```python
from build123d import *

# Parameters (mm, degrees)
SKETCH1_W                          = 101.6
SKETCH1_H                          = 31.75
BOSS_EXTRUDE1_DEPTH                = 3.175
CUT_EXTRUDE1_REACH                 = 55.6
SKETCH2_R                          = 1.63195
SKETCH2_R_2                        = 6.35
TAP_DRILL_FOR_6_32_TAP1_AT_2_COUNT = 2
TAP_DRILL_FOR_6_32_TAP1_AT_2_PITCH = 79.375
TAP_DRILL_FOR_6_32_TAP1_AT_3_COUNT = 2
TAP_DRILL_FOR_6_32_TAP1_AT_3_PITCH = 47.625


with BuildPart() as part:
    # Sketch1 → Boss-Extrude1 (new, symmetric)
    with BuildSketch(Plane(origin=(0, 0, 0), x_dir=(0, 0, -1), z_dir=(1, 0, 0))):
        Rectangle(SKETCH1_W, SKETCH1_H)
    extrude(amount=BOSS_EXTRUDE1_DEPTH, both=True)

    # Sketch2 → Cut-Extrude1 (cut, up to next)
    with BuildSketch(Plane(origin=(3.175, 0, 0), x_dir=(0, 0, -1), z_dir=(1, 0, 0)), mode=Mode.PRIVATE) as cut_extrude1_sk1:
        with Locations((-16.764, 8.255)):
            Circle(SKETCH2_R)
    cut_extrude1_tool1 = extrude(cut_extrude1_sk1.sketch, amount=-CUT_EXTRUDE1_REACH, mode=Mode.PRIVATE) & part.part
    # Sketch2 → Cut-Extrude1 (cut, up to next)
    with BuildSketch(Plane(origin=(3.175, 0, 0), x_dir=(0, 0, -1), z_dir=(1, 0, 0)), mode=Mode.PRIVATE) as cut_extrude1_sk2:
        with Locations((-16.764, -12.7)):
            Circle(SKETCH2_R)
    cut_extrude1_tool2 = extrude(cut_extrude1_sk2.sketch, amount=-CUT_EXTRUDE1_REACH, mode=Mode.PRIVATE) & part.part
    # Sketch2 → Cut-Extrude1 (cut, up to next)
    with BuildSketch(Plane(origin=(3.175, 0, 0), x_dir=(0, 0, -1), z_dir=(1, 0, 0)), mode=Mode.PRIVATE) as cut_extrude1_sk3:
        with Locations((40.005, -12.7)):
            Circle(SKETCH2_R)
    cut_extrude1_tool3 = extrude(cut_extrude1_sk3.sketch, amount=-CUT_EXTRUDE1_REACH, mode=Mode.PRIVATE) & part.part
    # Sketch2 → Cut-Extrude1 (cut, up to next)
    with BuildSketch(Plane(origin=(3.175, 0, 0), x_dir=(0, 0, -1), z_dir=(1, 0, 0)), mode=Mode.PRIVATE) as cut_extrude1_sk4:
        with Locations((40.005, 8.255)):
            Circle(SKETCH2_R)
    cut_extrude1_tool4 = extrude(cut_extrude1_sk4.sketch, amount=-CUT_EXTRUDE1_REACH, mode=Mode.PRIVATE) & part.part
    # Sketch2 → Cut-Extrude1 (cut, up to next)
    with BuildSketch(Plane(origin=(3.175, 0, 0), x_dir=(0, 0, -1), z_dir=(1, 0, 0)), mode=Mode.PRIVATE) as cut_extrude1_sk5:
        with Locations((-4.064, -2.2225)):
            Circle(SKETCH2_R_2)
    cut_extrude1_tool5 = extrude(cut_extrude1_sk5.sketch, amount=-CUT_EXTRUDE1_REACH, mode=Mode.PRIVATE) & part.part
    add(cut_extrude1_tool1.solids().sort_by_distance((3.175, 8.255, 16.764))[0], mode=Mode.SUBTRACT)
    add(cut_extrude1_tool2.solids().sort_by_distance((3.175, -12.7, 16.764))[0], mode=Mode.SUBTRACT)
    add(cut_extrude1_tool3.solids().sort_by_distance((3.175, -12.7, -40.005))[0], mode=Mode.SUBTRACT)
    add(cut_extrude1_tool4.solids().sort_by_distance((3.175, 8.255, -40.005))[0], mode=Mode.SUBTRACT)
    add(cut_extrude1_tool5.solids().sort_by_distance((3.175, -2.2225, 4.064))[0], mode=Mode.SUBTRACT)

    # Sketch5 → Tap Drill for #6-32 Tap1 (revolve, cut)
    with BuildSketch(Plane(origin=(0, 15.875, 44.45), x_dir=(0, 0, 1), z_dir=(1, 0, 0))):
        Polygon((0, 0), (0, 13.51269403), (1.35255, 12.7), (1.35255, 0), align=None)
    tap_drill_for_6_32_tap1 = revolve(axis=Axis((0, 22.225, 44.45), (0, -1, 0)), mode=Mode.SUBTRACT)

    # Tap Drill for #6-32 Tap1 at 2: Tap Drill for #6-32 Tap1 ×2
    with Locations(*[(0, 0, -i * TAP_DRILL_FOR_6_32_TAP1_AT_2_PITCH) for i in range(1, TAP_DRILL_FOR_6_32_TAP1_AT_2_COUNT)]):
        add(tap_drill_for_6_32_tap1, mode=Mode.SUBTRACT)

    # Tap Drill for #6-32 Tap1 at 3: Tap Drill for #6-32 Tap1 ×2
    with Locations(*[(0, 0, -i * TAP_DRILL_FOR_6_32_TAP1_AT_3_PITCH) for i in range(1, TAP_DRILL_FOR_6_32_TAP1_AT_3_COUNT)]):
        add(tap_drill_for_6_32_tap1, mode=Mode.SUBTRACT)

    # Mirror1: Tap Drill for #6-32 Tap1 across plane
    add(tap_drill_for_6_32_tap1.mirror(Plane.ZX), mode=Mode.SUBTRACT)

    # Mirror1 copy 1 sketch → Mirror1 copy 1 (revolve, cut)
    with BuildSketch(Plane(origin=(0, -15.875, -34.925), x_dir=(0, 0, 1), z_dir=(1, 0, 0))):
        Polygon((0, 0), (0, -13.51269403), (1.35255, -12.7), (1.35255, 0), align=None)
    revolve(axis=Axis((0, -22.225, -34.925), (0, -1, 0)), mode=Mode.SUBTRACT)

    # Mirror1 copy 2 sketch → Mirror1 copy 2 (revolve, cut)
    with BuildSketch(Plane(origin=(0, -15.875, -3.175), x_dir=(0, 0, 1), z_dir=(1, 0, 0))):
        Polygon((0, 0), (0, -13.51269403), (1.35255, -12.7), (1.35255, 0), align=None)
    revolve(axis=Axis((0, -22.225, -3.175), (0, -1, 0)), mode=Mode.SUBTRACT)


solid = part.part
```
Could you check a few things on this model? Use its own coordinates, in mm. A direction names the side the tool comes from. Coordinates: 2 decimals unless noted, no trailing zeros. Write each loop counter-clockwise with the first axis right and the second up, starting at its lowest first coordinate (ties: lowest second). Pieces come first, ordered by that corner, then holes. Notation, with made-up numbers: M -10,30.25 L 45,30.25 A17 cw 45,43.25 Z; hole C 45,17.25 d6. An arc over 180 degrees is marked long. Answer as CSV lines item,"result". Start each with the question number.
1) We'd pull the mould along Y, two halves only. Please class faces 4 (the cylindrical face through (0.04, -12.21, -41.56)), 5 (the cylindrical face through (0.044, 6.662, 17.118)), 6 (the flat face through (0, -15.875, 1)), 7 (the cylindrical face through (-0.059, -9.614, -4.526)): +Y half, -Y half, draft (parallel to the pull), parting line (faces both ways), or undercut.
2) For P1, Ø4, axis at y = 8.255, z = 16.764, coming from the -X side (3 decimals); P2, Ø2.5, axis at y = 8.255, z = -40.005, coming from the +X side; P3, Ø1.6, axis at x = 0, z = -34.925, coming from the +Y side; P4, Ø1.6, axis at x = 0, z = -3.175, coming from the -Y side, each with a flat end and sliding along its axis, tell me the tip position at first contact or that it passes through.
3) Please list where these lines run through material, in increasing order: line 1 (Z direction, x = 0, y = 11.5); line 2 (X direction, y = -10.25, z = 44.45) (3 decimals); line 3 (Z direction, x = -0.5, y = -6). Write a range as from..to.
4) I want a section at A-A, the plane y = -12.7. Please give me the cut outline in (x, z) (3 decimals).
5) I want a section at D-D, the plane y = 12. Please give me the cut outline in (x, z) (3 decimals), and give its area (3 significant figures).
6) I want a section at B-B, the plane y = -7. Please give me the cut outline in (x, z) (3 decimals), and give its area (3 significant figures).
7) I want a section at C-C, the plane x = 2.25. Give the number of separate pieces and of enclosed holes in the cut face, and give its area (3 significant figures).
8) For faces 1 (the cylindrical face through (0.518, 9.614, -1.926)), 2 (the cylindrical face through (-0.059, -9.614, -36.276)), 3 (the flat face through (0, 0, -50.8)), which set-ups out of +Z, -Z, +X, -X, +Y, -Y let a thin tool reach every point of the face, with its end or its side?
Data:
1,face 4,"undercut"
1,face 5,"undercut"
1,face 6,"-Y half"
1,face 7,"draft"
2,P1,"stops at x = -3.175"
2,P2,"passes through"
2,P3,"stops at y = 2.84"
2,P4,"stops at y = -2.84"
3,line 1,"z = -50.8..-36.28, -33.57..-4.53, -1.82..43.1, 45.8..50.8"
3,line 2,"x = -3.175..-1.353, 1.353..3.175"
3,line 3,"z = -50.8..-36.18, -33.67..-4.43, -1.92..-1.04, 9.17..43.19, 45.71..50.8"
4,outline,"M -3.175,-50.8 L 3.175,-50.8 L 3.175,-41.637 L -3.175,-41.637 Z; M -3.175,-38.373 L 3.175,-38.373 L 3.175,15.132 L -3.175,15.132 Z; M -3.175,18.396 L 3.175,18.396 L 3.175,50.8 L -3.175,50.8 Z; hole C 0,-34.925 d2.705; hole C 0,-3.175 d2.705; hole C 0,44.45 d2.705"
5,outline,"M -3.175,-50.8 L 3.175,-50.8 L 3.175,50.8 L -3.175,50.8 Z; hole C 0,-34.925 d2.705; hole C 0,-3.175 d2.705; hole C 0,44.45 d2.705"
5,area,"628 mm^2"
6,outline,"M -3.175,-50.8 L 3.175,-50.8 L 3.175,-0.119 L -3.175,-0.119 Z; M -3.175,8.247 L 3.175,8.247 L 3.175,50.8 L -3.175,50.8 Z; hole C 0,-34.925 d2.705; hole C 0,-3.175 d2.705; hole C 0,44.45 d2.705"
6,area,"575 mm^2"
7,separate pieces,"1"
7,enclosed holes,"5"
7,area,"3,070 mm^2"
8,face 1,"+Y"
8,face 2,"-Y"
8,face 3,"-Z, +X, -X, +Y, -Y"
